```python
from build123d import *

# Parameters (mm, degrees)
BUITENAFMETING_RECHTHOEK_W  = 90
BUITENAFMETING_RECHTHOEK_H  = 170
PLAAT_DEPTH                 = 4
TAND_HOR_W                  = 12.857142857
TAND_HOR_H                  = 4
TAND_BOVEN_DEPTH            = 5
TANDEN_PATROON_BOVEN_COUNT  = 3
TANDEN_PATROON_BOVEN_PITCH  = 25.714285714
TAND_VER_W                  = 4
TAND_VER_H                  = 24.285714285
TAND_LINKS_DEPTH            = 5
TANDEN_PATROON_LINKS_COUNT  = 3
TANDEN_PATROON_LINKS_PITCH  = 48.571428571
TAND_O_W                    = 12.857142857
TAND_O_H                    = 4
TAND_ONDER_DEPTH            = 5
TANDEN_PATROON_ONDER_COUNT  = 3
TANDEN_PATROON_ONDER_PITCH  = 25.714285714
TAND_R_W                    = 4
TAND_R_H                    = 24.285714285
TAND_RECHTS_DEPTH           = 5
TANDEN_PATROON_RECHTS_COUNT = 3
TANDEN_PATROON_RECHTS_PITCH = 48.571428571


with BuildPart() as part:
    # Buitenafmeting Rechthoek → Plaat (new body)
    with BuildSketch(Plane.XY):
        with Locations((45, 85)):
            Rectangle(BUITENAFMETING_RECHTHOEK_W, BUITENAFMETING_RECHTHOEK_H)
    extrude(amount=-PLAAT_DEPTH)

    # Tand Hor → Tand Boven (cut, through all)
    with BuildSketch(Plane.XY):
        with Locations((19.285714286, 168)):
            Rectangle(TAND_HOR_W, TAND_HOR_H)
    tand_boven = extrude(amount=-TAND_BOVEN_DEPTH, mode=Mode.SUBTRACT)

    # Tanden Patroon Boven: Tand Boven ×3
    with Locations(*[(i * TANDEN_PATROON_BOVEN_PITCH, 0, 0) for i in range(1, TANDEN_PATROON_BOVEN_COUNT)]):
        add(tand_boven, mode=Mode.SUBTRACT)

    # Tand Ver → Tand Links (cut, through all)
    with BuildSketch(Plane.XY):
        with Locations((2, 133.571428572)):
            Rectangle(TAND_VER_W, TAND_VER_H)
    tand_links = extrude(amount=-TAND_LINKS_DEPTH, mode=Mode.SUBTRACT)

    # Tanden Patroon Links: Tand Links ×3
    with Locations(*[(0, -i * TANDEN_PATROON_LINKS_PITCH, 0) for i in range(1, TANDEN_PATROON_LINKS_COUNT)]):
        add(tand_links, mode=Mode.SUBTRACT)

    # Tand O → Tand Onder (cut, through all)
    with BuildSketch(Plane.XY):
        with Locations((19.285714286, 2)):
            Rectangle(TAND_O_W, TAND_O_H)
    tand_onder = extrude(amount=-TAND_ONDER_DEPTH, mode=Mode.SUBTRACT)

    # Tanden Patroon Onder: Tand Onder ×3
    with Locations(*[(i * TANDEN_PATROON_ONDER_PITCH, 0, 0) for i in range(1, TANDEN_PATROON_ONDER_COUNT)]):
        add(tand_onder, mode=Mode.SUBTRACT)

    # Tand R → Tand Rechts (cut, through all)
    with BuildSketch(Plane.XY):
        with Locations((88, 133.571428572)):
            Rectangle(TAND_R_W, TAND_R_H)
    tand_rechts = extrude(amount=-TAND_RECHTS_DEPTH, mode=Mode.SUBTRACT)

    # Tanden Patroon Rechts: Tand Rechts ×3
    with Locations(*[(0, -i * TANDEN_PATROON_RECHTS_PITCH, 0) for i in range(1, TANDEN_PATROON_RECHTS_COUNT)]):
        add(tand_rechts, mode=Mode.SUBTRACT)


solid = part.part
```
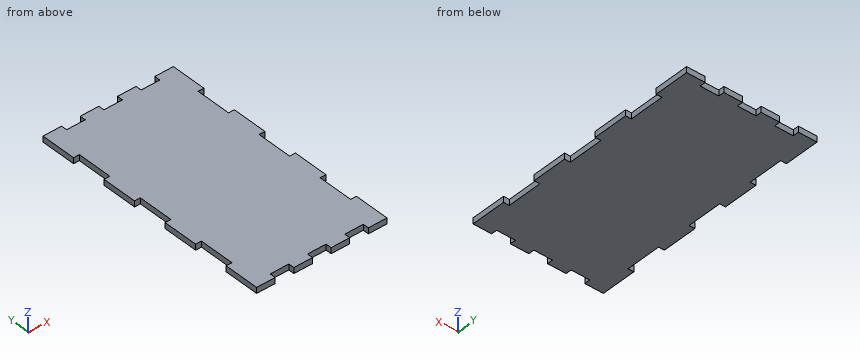
Model file for the job. Use its own axes, mm. Coordinates: 2 decimals unless noted, no trailing zeros. Order: outer loops, then holes, each group sorted by start corner. A loop starts at its lowest first (then second) coordinate and runs counter-clockwise, first axis right, second up. Notation, with made-up numbers: M 12.25,79 L 64.25,79 A21 ccw 64.25,88 Z; hole C 46.25,79 d7. An arc over 180 degrees is marked long. Answer as CSV lines item,"result".
(1) Band-saw the part on A-A, the plane y = 87. List the corners of the cut face in (x, z), then the cut area to 3 significant figures.
Geometry says:
outline,"M 4,-4 L 86,-4 L 86,0 L 4,0 Z"
area,"328 mm2"
(2) Flat gauge pins, fed straight in: pin 1 (1.2 mm diameter, centred on y = 86, z = -1.5, fed in from -X); pin 2 (2 mm diameter, centred on x = 20, z = -2.5, fed in from -Y); pin 3 (1.2 mm diameter, centred on x = 72, z = -1, fed in from +Y). Where does each tip first touch, or does it go through?
Geometry says:
pin 1,"stops at x = 4"
pin 2,"stops at y = 4"
pin 3,"stops at y = 166"
(3) Wall check: line 1 along Y through (x, z) = (67, -1.75); line 2 along X through (y, z) = (82, -2.35). Give the ranges that are in metal, low to high.
Geometry says:
line 1,"y = 4 to 166"
line 2,"x = 4 to 86"
(4) Band-saw the part on B-B, the plane x = 43.5. List the corners of the cut face in (y, z).
Geometry says:
outline,"M 4,-4 L 166,-4 L 166,0 L 4,0 Z"
